Input: dimensioned drawing with shaded views. Units: mm. Origin: part minimum x, y, z. A direction names the side the tool comes from. Round coordinates to 2 decimals unless told otherwise and drop trailing zeros. Loops run counter-clockwise (first coordinate to the right, second up) from the corner with the lowest first, then second, coordinate; pieces in that order, holes last. Notation, with made-up numbers: M -27.5,77 L 0.5,77 A13 cw 0.5,96 Z; hole C -1,66.5 d11. An arc over 180 degrees is marked long. Put each result on its own line as item: value. Start each with the question number.
1) Line query: probe 1 along Z at (x, y) = (11, 3.5); probe 2 along Y at (x, z) = (12.5, 6); probe 3 along Z at (x, y) = (7.05, 10). Output: solid intervals per line, ascending.
2) Section C-C on z = 18.5. Output: boundary loops of the cut face in (x, y).
3) Pin query (flat end, axial travel): pin 1 (8 mm diameter, centred on y = 10, z = 6, fed in from +X); pin 2 (4 mm diameter, centred on x = 11, z = 15, fed in from +Y); pin 3 (10 mm diameter, centred on y = 4.5, z = 7.5, fed in from -X). Return the tip coordinate at first contact, or that it passes through.
4) Section B-B on x = 10.75. Output: boundary loops of the cut face in (y, z).
5) Reachability of the marked faces 1, 2, 3 and 4 from +Z, -Z, +X, -X, +Y, -Y: full face, straight path, thin tool, end or side. Return the list, or none.
6) Section A-A on z = 15. Output: boundary loops of the cut face in (x, y).
7) Section D-D on y = 16. Output: boundary loops of the cut face in (x, z).
8) Draft query along X for the marked faces 5, 6, 7 and 8. Return one class per face: +X half, -X half, draft (parallel to the pull), parting line (faces both ways), or undercut.
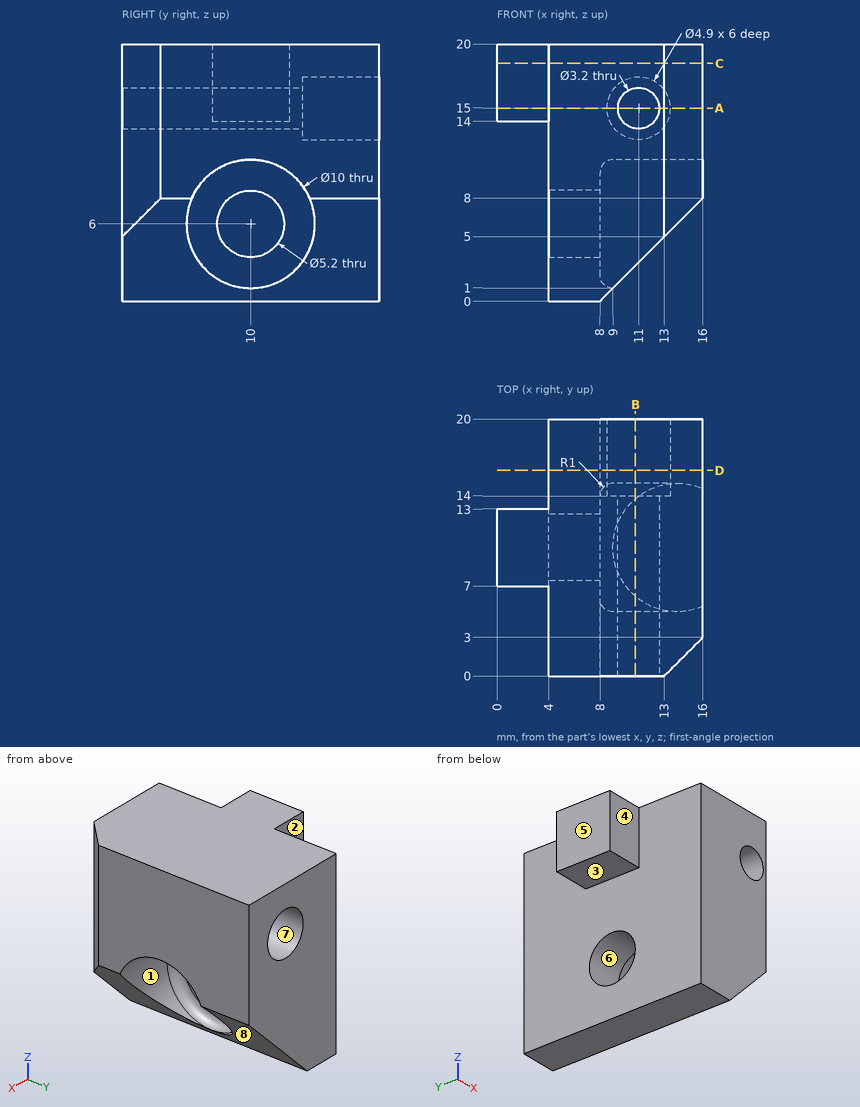
Geometry results:
1. probe 1: z = 3 to 13.4, 16.6 to 20
1. probe 2: y = 0 to 5, 15 to 20
1. probe 3: z = 0 to 3.4, 8.6 to 20
2. outline: M 0,7 L 4,7 L 4,0 L 13,0 L 16,3 L 16,20 L 4,20 L 4,13 L 0,13 Z
3. pin 1: stops at x = 8
3. pin 2: stops at y = 14
3. pin 3: stops at x = 4
4. outline: M 0,2.75 L 6.2,2.75 A5 cw long 13.8,2.75 L 20,2.75 L 20,12.56 L 14,12.56 L 14,13.42 L 0,13.42 Z; M 0,16.58 L 14,16.58 L 14,17.44 L 20,17.44 L 20,20 L 0,20 Z
5. face 1: +X
5. face 2: +Z, -Z, -X, +Y
5. face 3: -Z, -X, +Y, -Y
5. face 4: +Z, -Z, -X, -Y
6. outline: M 0,7 L 4,7 L 4,0 L 9.4,0 L 9.4,14 L 8.55,14 L 8.55,20 L 4,20 L 4,13 L 0,13 Z; M 12.6,0 L 13,0 L 16,3 L 16,20 L 13.45,20 L 13.45,14 L 12.6,14 Z
7. outline: M 4,0 L 8,0 L 16,8 L 16,20 L 4,20 Z; hole C 11,15 d4.9
8. face 5: -X half
8. face 6: draft
8. face 7: undercut
8. face 8: +X half
